The model under review builds one solid part; all positions refer to its coordinate system, in mm. A direction names the side the tool comes from. Give positions to 0.01 mm unless a question says otherwise; leave off trailing zeros. Order: outer loops, then holes, each group sorted by start corner. A loop starts at its lowest first (then second) coordinate and runs counter-clockwise, first axis right, second up. Notation, with made-up numbers: (3, 18) - (31, 18) arc R33 ccw to (31, 47) - close; hole circle Ø8 at (85.5, 30.25). An arc over 180 degrees is marked (long way). Use CSV: the item, a comma, the result in double quotes. Start each with the question number.
```python
from build123d import *

# Parameters (mm, degrees)
F1_DEPTH = 80
F2_DEPTH = 170
F3_DEPTH = 135


with BuildPart() as f1:
    # F0 (on Top) → F1 (new body)
    with BuildSketch(Plane.XY):
        with BuildLine():
            Line((41.930038482, 39.4312292337), (41.930038482, 55))
            Line((41.930038482, 55), (-13.9003656805, 55))
            Line((-13.9003656805, 55), (-13.9003656805, 39.4312292337))
            Line((-13.9003656805, 39.4312292337), (-72, 39.4312292337))
            Line((-72, 39.4312292337), (-72, -55))
            Line((-72, -55), (-5.7156333832, -55))
            ThreePointArc((-5.7156333832, -55), (-6.1417465241, 24.75499425), (63, -15))
            ThreePointArc((63, -15), (56.75499425, -38.1417465241), (39.7156333832, -55))
            Line((39.7156333832, -55), (72, -55))
            Line((72, -55), (72, 39.4312292337))
            Line((72, 39.4312292337), (41.930038482, 39.4312292337))
        make_face()
    extrude(amount=F1_DEPTH)

    # F0 (on Top) → F2 (join)
    with BuildSketch(Plane.XY):
        with BuildLine():
            ThreePointArc((-5.7156333832, -55), (17, -61), (39.7156333832, -55))
            Line((39.7156333832, -55), (-5.7156333832, -55))
        make_face()
        with BuildLine():
            Line((-5.7156333832, -55), (39.7156333832, -55))
            ThreePointArc((39.7156333832, -55), (56.75499425, -38.1417465241), (63, -15))
            ThreePointArc((63, -15), (-6.1417465241, 24.75499425), (-5.7156333832, -55))
        make_face()
    extrude(amount=F2_DEPTH)

    # F0 (on Top) → F3 (cut)
    with BuildSketch(Plane.XY):
        with BuildLine():
            ThreePointArc((-5.7156333832, -55), (17, -61), (39.7156333832, -55))
            Line((39.7156333832, -55), (-5.7156333832, -55))
        make_face()
    extrude(amount=F3_DEPTH, mode=Mode.SUBTRACT)


solid = f1.part
```
1. Consider section C-C (y = 44.5). Give the boundary of the cut face in (x, z).
2. Consider section B-B (x = 17). Give the boundary of the cut face in (y, z), and give its area (4 significant figures).
3. Clearance check with flat-ended pins moving along their axes: pin 1 (10 mm diameter, centred on y = -7, z = 117.5, fed in from +X); pin 2 (1 mm diameter, centred on x = -27.5, z = 40.5, fed in from +Y); pin 3 (1 mm diameter, centred on x = 27, y = 1, fed in from -Z); pin 4 (8 mm diameter, centred on y = 50, z = 58.5, fed in from +X). State where each tip first meets the part, or that it passes through.
4. Tool access review of faces 1 (the face through (41.93, 47, 39)), 2 (the face through (-43, 39.431, 39)), 3 (the face through (-1, 1, 0)), 4 (the face through (17, -57, 135)), 5 (the face through (14, 55, 39)): name each direction out of +Z, -Z, +X, -X, +Y, -Y from which nothing blocks a thin tool from reaching the whole face with its end or side.
5. Consider section D-D (x = -50). Give the boundary of the cut face in (y, z).
6. To check wall thickness, follow L1, parallel to Y at x = -1, z = 25; L2, parallel to Y at x = 15, z = 111; L3, parallel to Z at x = 12.5, y = 34.5. State the ranges of each line that lie inside material, in increasing order. Write a range as [from, to].
7. Consider section A-A (z = 53). Give the boundary of the cut face in (x, y), and give its area (3 significant figures).
Answers follow:
1,outline,"(-13.9, 0) - (41.93, 0) - (41.93, 80) - (-13.9, 80) - close"
2,outline,"(-61, 135) - (-55, 135) - (-55, 0) - (55, 0) - (55, 80) - (31, 80) - (31, 170) - (-61, 170) - close"
2,area,"16,750 mm^2"
3,pin 1,"stops at x = 62.9"
3,pin 2,"stops at y = 39.43"
3,pin 3,"stops at z = 0"
3,pin 4,"stops at x = 41.93"
4,face 1,"+Z, -Z, +X, +Y"
4,face 2,"+Z, -Z, -X, +Y"
4,face 3,"-Z, +X, -X, +Y, -Y"
4,face 4,"-Z, +X, -X, -Y"
4,face 5,"+Z, -Z, +X, -X, +Y"
5,outline,"(-55, 0) - (39.43, 0) - (39.43, 80) - (-55, 80) - close"
6,L1,"y = [-55, 55]"
6,L2,"y = [-55, 30.96]"
6,L3,"z = [0, 80]"
7,outline,"(-72, -55) - (72, -55) - (72, 39.43) - (41.93, 39.43) - (41.93, 55) - (-13.9, 55) - (-13.9, 39.43) - (-72, 39.43) - close"
7,area,"14,500 mm^2"
